from build123d import *

# Parameters (mm, degrees)
SKETCH1_W           = 50.8
SKETCH1_H           = 248.000519746
SKETCH1_R           = 4.0000047
SKETCH1_R_2         = 15.113
BOSS_EXTRUDE1_DEPTH = 19.05
CUT_EXTRUDE1_REACH  = 137.35
SKETCH3_R           = 2.0828
CUT_EXTRUDE2_REACH  = 130
FILLET2_R           = 3.175
FILLET3_R           = 3.175
CUT_EXTRUDE3_REACH  = 124.668
SKETCH8_R           = 1.500000048
CUT_EXTRUDE4_REACH  = 124.668
SKETCH12_W          = 3.81
SKETCH12_H          = 6.719538638
BOSS_EXTRUDE3_DEPTH = 19.05
SKETCH14_R          = 1.500000048
CUT_EXTRUDE5_DEPTH  = 109.729869862
BOSS_EXTRUDE5_DEPTH = 19.05
FILLET4_R           = 0.635


with BuildPart() as part:
    # Sketch1 → Boss-Extrude1 (new body)
    with BuildSketch(Plane.XY):
        Rectangle(SKETCH1_W, SKETCH1_H)
        with Locations(Location((0, -98.600259873, 0), (0, 0, 180))):
            Circle(SKETCH1_R, mode=Mode.SUBTRACT)
        with Locations(Location((0, 79.550259873, 0), (0, 0, 180))):
            Circle(SKETCH1_R_2, mode=Mode.SUBTRACT)
    extrude(amount=BOSS_EXTRUDE1_DEPTH)

    # Sketch3 → Cut-Extrude1 (cut, up to next)
    with BuildSketch(Plane(origin=(25.4, 0, 0), x_dir=(0, 0, -1), z_dir=(1, 0, 0)), mode=Mode.PRIVATE) as cut_extrude1_sk1:
        with Locations((-9.525, 99.870259873)):
            Circle(SKETCH3_R)
    cut_extrude1_tool1 = extrude(cut_extrude1_sk1.sketch, amount=-CUT_EXTRUDE1_REACH, mode=Mode.PRIVATE) & part.part
    add(cut_extrude1_tool1.solids().sort_by_distance((25.4, 99.87026, 9.525))[0], mode=Mode.SUBTRACT)

    # Sketch4 → Cut-Extrude2 (cut, up to next)
    with BuildSketch(Plane.XY.offset(19.05), mode=Mode.PRIVATE) as cut_extrude2_sk1:
        with BuildLine():
            Line((25.4, -124.000259873), (25.4, 49.070259873))
            Line((25.4, 49.070259873), (11.078372462, -99.666975439))
            ThreePointArc((11.078372462, -99.666975439), (-0.533972701, -109.7170531), (-11.129609989, -98.600259873))
            Line((-11.129609989, -98.600259873), (-21.277335587, 77.084025085))
            ThreePointArc((-21.277335587, 77.084025085), (-21.384145342, 78.315087136), (-21.419788134, 79.550259873))
            ThreePointArc((-21.419788134, 79.550259873), (-19.121183474, 89.203635773), (-12.718706155, 96.785161597))
            ThreePointArc((-12.718706155, 96.785161597), (-12.44619853, 96.982972395), (-12.170614954, 97.176474877))
            Line((-12.170614954, 97.176474877), (16.725657691, 117.807156743))
            Line((16.725657691, 117.807156743), (25.4, 124.000259873))
            Line((25.4, 124.000259873), (-25.4, 124.000259873))
            Line((-25.4, 124.000259873), (-25.4, -124.000259873))
            Line((-25.4, -124.000259873), (25.4, -124.000259873))
        make_face()
    cut_extrude2_tool1 = extrude(cut_extrude2_sk1.sketch, amount=-CUT_EXTRUDE2_REACH, mode=Mode.PRIVATE) & part.part
    # Sketch4 → Cut-Extrude2 (cut, up to next)
    with BuildSketch(Plane.XY.offset(19.05), mode=Mode.PRIVATE) as cut_extrude2_sk2:
        with BuildLine():
            ThreePointArc((16.725657691, 117.807156743), (22.540648101, 117.636552978), (25.4, 112.570259873))
            Line((25.4, 112.570259873), (25.4, 124.000259873))
            Line((25.4, 124.000259873), (16.725657691, 117.807156743))
        make_face()
    cut_extrude2_tool2 = extrude(cut_extrude2_sk2.sketch, amount=-CUT_EXTRUDE2_REACH, mode=Mode.PRIVATE) & part.part
    # Sketch4 → Cut-Extrude2 (cut, up to next)
    with BuildSketch(Plane.XY.offset(19.05), mode=Mode.PRIVATE) as cut_extrude2_sk3:
        with BuildLine():
            ThreePointArc((5.292525145, -81.359808555), (0.293269038, -87.451084718), (-5.679257035, -82.310545911))
            Line((-5.679257035, -82.310545911), (-14.092209721, 63.41901848))
            ThreePointArc((-14.092209721, 63.41901848), (5.243866663, 58.78227523), (20.060972069, 72.042615545))
            Line((20.060972069, 72.042615545), (5.292525145, -81.359808555))
        make_face()
    cut_extrude2_tool3 = extrude(cut_extrude2_sk3.sketch, amount=-CUT_EXTRUDE2_REACH, mode=Mode.PRIVATE) & part.part
    add(cut_extrude2_tool1.solids().sort_by_distance((22.8685, -37.465, 19.05))[0], mode=Mode.SUBTRACT)
    add(cut_extrude2_tool2.solids().sort_by_distance((23.100822, 119.489273, 19.05))[0], mode=Mode.SUBTRACT)
    add(cut_extrude2_tool3.solids().sort_by_distance((1.517355, 0.15341, 19.05))[0], mode=Mode.SUBTRACT)

    # Fillet2
    fillet2_edges = [part.edges().sort_by_distance(p)[0] for p in [
        (-14.092209721, 63.41901848, 9.525),
    ]]
    fillet(fillet2_edges, radius=FILLET2_R)

    # Fillet3
    fillet3_edges = [part.edges().sort_by_distance(p)[0] for p in [
        (20.060972069, 72.042615545, 9.525),
    ]]
    fillet(fillet3_edges, radius=FILLET3_R)

    # Sketch8 → Cut-Extrude3 (cut, up to next)
    with BuildSketch(Plane(origin=(0, 0, 0), x_dir=(1, 0, 0), z_dir=(0, 1, 0)), mode=Mode.PRIVATE) as cut_extrude3_sk1:
        with Locations(Location((0, -9.525, 0), (0, 0, 270))):
            Circle(SKETCH8_R)
    cut_extrude3_tool1 = extrude(cut_extrude3_sk1.sketch, amount=-CUT_EXTRUDE3_REACH, mode=Mode.PRIVATE) & part.part
    add(cut_extrude3_tool1.solids().sort_by_distance((0, 0, 9.525))[0], mode=Mode.SUBTRACT)
    add(cut_extrude3_tool1.solids().sort_by_distance((0, 0, 9.525))[1], mode=Mode.SUBTRACT)

    # Sketch9 → Cut-Extrude4 (cut, up to next)
    with BuildSketch(Plane.XY.offset(19.05), mode=Mode.PRIVATE) as cut_extrude4_sk1:
        with BuildLine():
            Line((21.59, 93.837951404), (21.59, 110.430718326))
            ThreePointArc((21.59, 110.430718326), (19.868129262, 113.2536672), (16.570132064, 113.014724382))
            Line((16.570132064, 113.014724382), (4.664459855, 104.514592245))
            ThreePointArc((4.664459855, 104.514592245), (3.379291217, 101.398142719), (5.622621351, 98.88191817))
            ThreePointArc((5.622621351, 98.88191817), (11.317754993, 96.200644412), (15.90649227, 91.891669316))
            ThreePointArc((15.90649227, 91.891669316), (19.443618723, 90.834192339), (21.59, 93.837951404))
        make_face()
    cut_extrude4_tool1 = extrude(cut_extrude4_sk1.sketch, amount=-CUT_EXTRUDE4_REACH, mode=Mode.PRIVATE) & part.part
    add(cut_extrude4_tool1.solids().sort_by_distance((14.719372, 102.332166, 19.05))[0], mode=Mode.SUBTRACT)

    # Sketch12 → Boss-Extrude3 (add)
    with BuildSketch(Plane.XY.offset(19.05)):
        with Locations((0, -106.370100543)):
            Rectangle(SKETCH12_W, SKETCH12_H)
    extrude(amount=-BOSS_EXTRUDE3_DEPTH)

    # Sketch14 → Cut-Extrude5 (cut)
    with BuildSketch(Plane(origin=(0, 0, 0), x_dir=(1, 0, 0), z_dir=(0, 1, 0))):
        with Locations(Location((0, -9.525, 0), (0, 0, 270))):
            Circle(SKETCH14_R)
    extrude(amount=-CUT_EXTRUDE5_DEPTH, mode=Mode.SUBTRACT)

    # Sketch17 → Boss-Extrude5 (add)
    with BuildSketch(Plane.XY.offset(19.05)):
        Polygon((-14.392423467, -42.112227423), (-13.782717735, -52.66786519), (-18.505869398, -50.292966075), align=None)
    extrude(amount=-BOSS_EXTRUDE5_DEPTH)

    # Fillet4
    fillet4_edges = [part.edges().sort_by_distance(p)[0] for p in [
        (-18.505869398, -50.292966075, 9.525),
    ]]
    fillet(fillet4_edges, radius=FILLET4_R)


solid = part.part
Source: CAD feature listing. Evaluate the final solid. Frame: model axes, mm. A direction names the side the tool comes from. Round coordinates to 2 decimals unless told otherwise and drop trailing zeros. Order: outer loops, then holes, each group sorted by start corner. A loop starts at its lowest first (then second) coordinate and runs counter-clockwise, first axis right, second up. Notation, with made-up numbers: (47.5, -27) - (85.5, -27) arc R15 ccw to (85.5, -10) - close; hole circle Ø6 at (-33, 18.5). An arc over 180 degrees is marked (long way). Use a Markdown table: item, result. Add a question column.
1. Set-up query: faces 1 (the cylindrical face through (8.23, -106.09, 9.66)), 2 (the flat face through (-16.33, -45.97, 9.66)), 3 (the cylindrical face through (19.91, 113.23, 9.66)). Return all of +Z, -Z, +X, -X, +Y, -Y with unobstructed straight access to the full face (end or side cutting, diameter ignored); none if empty.
2. First-contact query: pin 1 (5 mm diameter, centred on y = -37, z = 9.5, fed in from -X); pin 2 (5 mm diameter, centred on y = 99.87, z = 9.52, fed in from -X); pin 3 (4 mm diameter, centred on x = 0, z = 9.525, fed in from +Y); pin 4 (10.5 mm diameter, centred on x = 0, y = -98.6, fed in from +Z). Flat tips, straight axial feed; report the tip coordinate or a pass-through.
3. Mould query, pull axis Z, two halves, no side actions, for faces 4 (the cylindrical face through (23.522, 101.935, 9.796)), 5 (the cylindrical face through (-1.289, 97.837, 9.977)), 6 (the flat face through (16, 13, 0)), 7 (the flat face through (1.7, -109.73, 9.7)). Classes: +Z half, -Z half, draft (parallel to the pull), parting line (faces both ways), or undercut.
4. Section query C-C (y = 82). Return the cut outline in (x, z), then the cut area to 3 significant figures.
5. Line query: probe 1 along X at (y, z) = (92, 9.75); probe 2 along Z at (x, y) = (0, -107.5) (3 decimals); probe 3 along Y at (x, z) = (1.5, 4). Output: solid intervals per line, ascending.
6. Section query B-B (z = 16.25). Give the number of separate pieces and of enclosed holes in the cut face, then the cut area to 3 significant figures.
7. Section query A-A (y = -19). Return the cut outline in (x, z).
Derived:
| question | item | result |
|---|---|---|
| 1 | face 1 | +Z, -Z, +X, -Y |
| 1 | face 2 | +Z, -Z, -X |
| 1 | face 3 | +Z, -Z |
| 2 | pin 1 | x = -14.83 |
| 2 | pin 2 | x = -11.9 |
| 2 | pin 3 | y = 107.29 |
| 2 | pin 4 | z = 19.05 |
| 3 | face 4 | undercut |
| 3 | face 5 | undercut |
| 3 | face 6 | -Z half |
| 3 | face 7 | draft |
| 4 | outline | (-21.28, 0) - (-14.91, 0) - (-14.91, 19.05) - (-21.28, 19.05) - close; (14.91, 0) - (25.4, 0) - (25.4, 19.05) - (14.91, 19.05) - close |
| 4 | area | 321 mm2 |
| 5 | probe 1 | -17.43 to -8.57, 8.57 to 15.82, 21 to 25.4 |
| 5 | probe 2 | 0 to 8.025, 11.025 to 19.05 |
| 5 | probe 3 | -109.73 to -102.31, -94.89 to -87.21, 58.18 to 64.51, 94.59 to 106.94 |
| 6 | separate pieces | 1 |
| 6 | enclosed holes | 4 |
| 6 | area | 3,660 mm2 |
| 7 | outline | (-15.73, 0) - (-9.33, 0) - (-9.33, 19.05) - (-15.73, 19.05) - close; (11.3, 0) - (18.85, 0) - (18.85, 19.05) - (11.3, 19.05) - close |
